Study the drawing (mm; zero at the part's minimum x, y, z) and answer. Round coordinates to 2 decimals unless told otherwise and drop trailing zeros. Write each loop counter-clockwise with the first axis right and the second up, starting at its lowest first coordinate (ties: lowest second). Pieces come first, ordered by that corner, then holes.
(1) A cutting plane is placed at A-A, the plane y = 15. Give the vertices of the cut face in (x, z), and give its area (3 significant figures).
(2) A cutting plane is placed at B-B, the plane z = 24. Give the vertices of the cut face in (x, y), and give its area (3 significant figures).
(3) Each of these flat-tipped pins is pushed along its axis until it touches: pin 1 Ø1 at (x, z) = (2.5, 16.5) entering from +Y; pin 2 Ø8 at (y, z) = (15, 42.25) entering from +X; pin 3 Ø1.5 at (x, z) = (1.5, 30.5) entering from +Y. Where does it stop, or does it pass through?
(4) The mould has two halves that part along Z. Classify the marked faces 1, 2 and 3: +Z half, -Z half, draft (parallel to the pull), parting line (faces both ways), or undercut.
(5) Find the intervals of material crossed by probe 1 along Z at (x, y) = (3.6, 16); probe 2 along Y at (x, z) = (2.2, 24); probe 3 along Y at (x, z) = (3.5, 13) (1 decimal), in increasing order.
(6) A cutting plane is placed at C-C, the plane x = 2.25. Give the vertices of the cut face in (y, z).
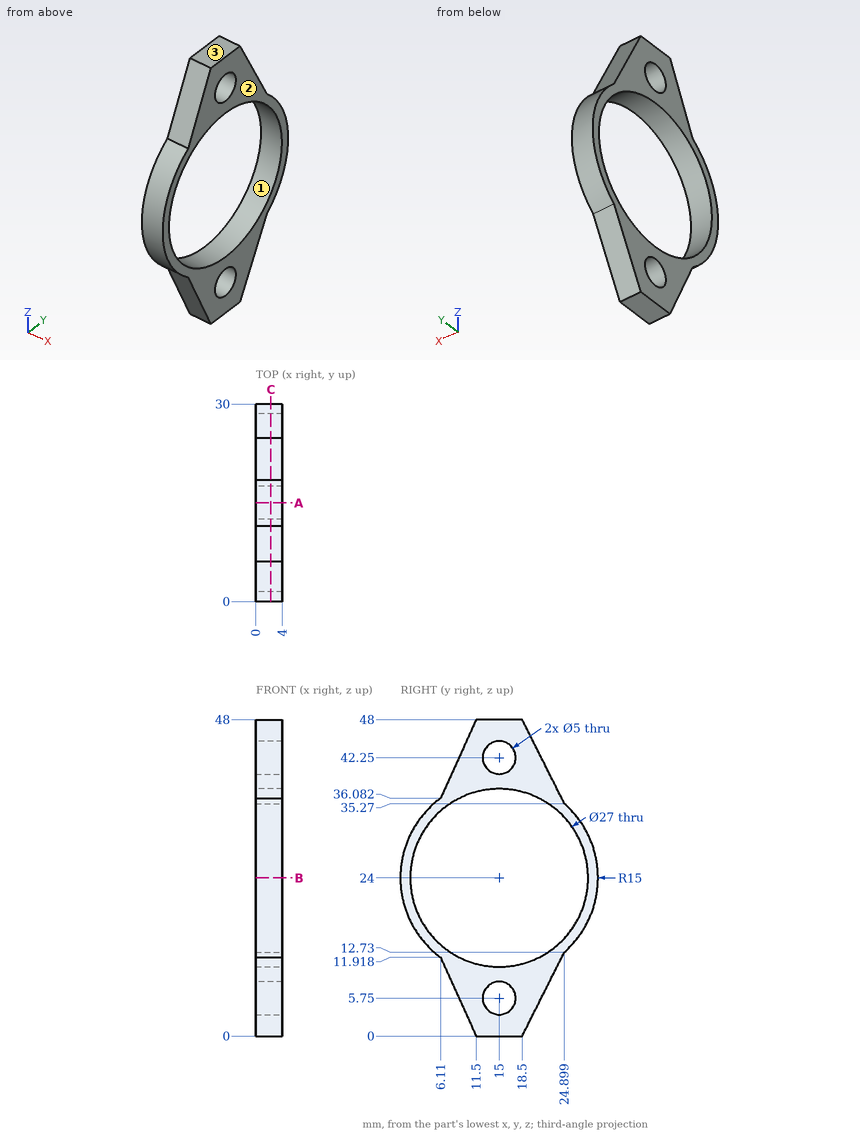
Solutions:
1. outline: (0, 0) - (4, 0) - (4, 3.25) - (0, 3.25) - close; (0, 8.25) - (4, 8.25) - (4, 10.5) - (0, 10.5) - close; (0, 37.5) - (4, 37.5) - (4, 39.75) - (0, 39.75) - close; (0, 44.75) - (4, 44.75) - (4, 48) - (0, 48) - close
1. area: 44.0 mm2
2. outline: (0, 0) - (4, 0) - (4, 1.5) - (0, 1.5) - close; (0, 28.5) - (4, 28.5) - (4, 30) - (0, 30) - close
2. area: 12.0 mm2
3. pin 1: stops at y = 28.27
3. pin 2: stops at x = 4
3. pin 3: stops at y = 28.85
4. face 1: undercut
4. face 2: draft
4. face 3: +Z half
5. probe 1: z = 0 to 3.46, 8.04 to 10.54, 37.46 to 39.96, 44.54 to 48
5. probe 2: y = 0 to 1.5, 28.5 to 30
5. probe 3: y = 4.8 to 7.2, 22.8 to 25.2
6. outline: (6.11, 11.92) - (11.5, 0) - (18.5, 0) - (24.9, 12.73) arc R15 ccw to (24.9, 35.27) - (18.5, 48) - (11.5, 48) - (6.11, 36.08) arc R15 ccw to start; hole circle Ø27 at (15, 24); hole circle Ø5 at (15, 5.75); hole circle Ø5 at (15, 42.25)
